For this review, take the finished solid that the model builds, in its own axes (mm). Face numbers are marked on the shaded views. Coordinates: 2 decimals unless noted, no trailing zeros. Loops run counter-clockwise (first coordinate to the right, second up) from the corner with the lowest first, then second, coordinate; pieces in that order, holes last. Notation, with made-up numbers: M -30.5,-21 L 1.5,-21 A28 ccw 1.5,1 Z; hole C 46.25,72.25 d5. An arc over 180 degrees is marked long. Put each result on its own line as item: value.
```python
from build123d import *
from OCP.BRepFilletAPI import BRepFilletAPI_MakeChamfer

# Parameters (mm, degrees)
SKETCH_1_R          = 2.05
EXTRUDE_1_DEPTH     = 10
CHAMFER_1_SIZE      = 4
CHAMFER_1_SIZE2     = 5.656854249
CHAMFER_1_SIZE2_2   = 3.265986324
SKETCH_2_R          = 12.5
CUT_EXTRUDE_1_DEPTH = 56.856960175
FILLET_1_R          = 2.5


with BuildPart() as part:
    # 草图1 → 凸台-拉伸1 (new, symmetric)
    with BuildSketch(Plane.XY):
        Polygon((-13.032253728, 10), (1.437002663, -44), (17.110272543, -44), (28, -10), (28, 10), align=None)
        Circle(SKETCH_1_R, mode=Mode.SUBTRACT)
        with Locations((20, 0)):
            Circle(SKETCH_1_R, mode=Mode.SUBTRACT)
        with Locations((9.110272543, -34)):
            Circle(SKETCH_1_R, mode=Mode.SUBTRACT)
    extrude(amount=EXTRUDE_1_DEPTH, both=True)

    # 倒角1: one chamfer whose edges measure the first distance from different faces: ONE call of the kernel's chamfer builder (chamfer() names one face for all edges)
    chamfer_1_edges_1 = [part.edges().sort_by_distance(p)[0] for p in [
        (1.437002663, -44, 0),
    ]]
    chamfer_1_side_1 = [part.faces().sort_by_distance(p)[0] for p in [
        (-5.797625533, -17, 0),
    ]]
    chamfer_1_edges_2 = [part.edges().sort_by_distance(p)[0] for p in [
        (-13.032253728, 10, 0),
    ]]
    chamfer_1_side_2 = [part.faces().sort_by_distance(p)[0] for p in [
        (-5.797625533, -17, 0),
    ]]
    chamfer_1_edges_3 = [part.edges().sort_by_distance(p)[0] for p in [
        (28, 10, 0),
    ]]
    chamfer_1 = BRepFilletAPI_MakeChamfer(part.part.solid().wrapped)
    for e in chamfer_1_edges_1:
        chamfer_1.Add(CHAMFER_1_SIZE, CHAMFER_1_SIZE2, e.wrapped, chamfer_1_side_1[0].wrapped)  # the first distance lies on this face
    for e in chamfer_1_edges_2:
        chamfer_1.Add(CHAMFER_1_SIZE, CHAMFER_1_SIZE2_2, e.wrapped, chamfer_1_side_2[0].wrapped)  # the first distance lies on this face
    for e in chamfer_1_edges_3:
        chamfer_1.Add(CHAMFER_1_SIZE, e.wrapped)
    add(Compound.cast(chamfer_1.Shape()), mode=Mode.REPLACE)

    # 草图2 → 切除-拉伸1 (cut, through all)
    with BuildSketch(Plane.XY.offset(10)):
        with Locations((29.991739345, -25.62060001)):
            Circle(SKETCH_2_R)
    extrude(amount=-CUT_EXTRUDE_1_DEPTH, mode=Mode.SUBTRACT)

    # 圆角1
    fillet_1_edges = [part.edges().sort_by_distance(p)[0] for p in [
        (-9.766267405, 10, 0),
        (24, 10, 0),
        (28, 6, 0),
        (0.401726482, -40.136296695, 0),
        (-11.996977548, 6.136296695, 0),
        (7.093856912, -44, 0),
        (26.873983288, -13.515658987, 0),
        (20.421472383, -33.661743602, 0),
        (17.110272543, -44, 0),
        (28, -10, 0),
    ]]
    fillet(fillet_1_edges, radius=FILLET_1_R)


solid = part.part
```
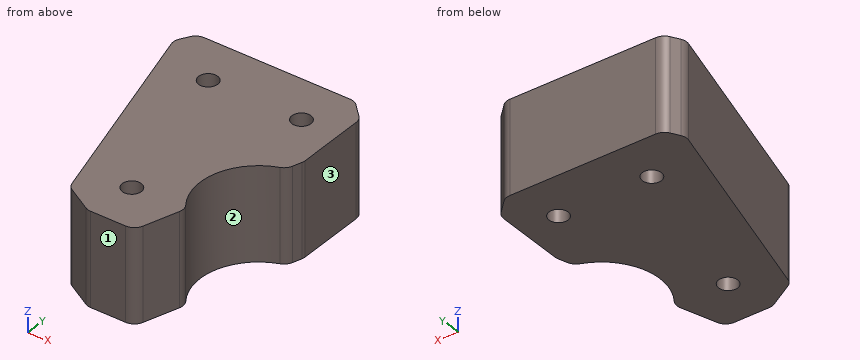
(1) Add section A-A (z = -2.25). Write out the cut boundary in (x, y), plus the area to 3 significant figures.
Determined:
outline: M -11.73,5.14 L 0.13,-39.14 A2.5 ccw 1.3,-40.65 L 6.51,-43.67 A2.5 ccw 7.76,-44 L 15.29,-44 A2.5 ccw 17.67,-42.26 L 20.02,-34.9 A2.5 ccw 19.7,-32.72 A12.5 cw 25.74,-13.87 A2.5 ccw 27.27,-12.28 L 27.88,-10.37 A2.5 ccw 28,-9.61 L 28,4.96 A2.5 ccw 27.27,6.73 L 24.73,9.27 A2.5 ccw 22.96,10 L -8.32,10 A2.5 ccw -10.49,8.75 L -11.48,7.03 A2.5 ccw Z; hole C 0,0 d4.1; hole C 9.11,-34 d4.1; hole C 20,0 d4.1
area: 1,490 mm^2
(2) Add section B-B (y = -1). Write out the cut boundary in (x, z).
Determined:
outline: M -10.08,-10 L -1.79,-10 L -1.79,10 L -10.08,10 Z; M 1.79,-10 L 18.21,-10 L 18.21,10 L 1.79,10 Z; M 21.79,-10 L 28,-10 L 28,10 L 21.79,10 Z
(3) Wall thickness on line 1 along Y through (x, z) = (9, -0.75); line 2 along X through (y, z) = (1, -6.75); line 3 along Y through (x, z) = (3, -3.5): over which ranges is each line inside the solid? List them lowest first. Write a range as [from, to].
Determined:
line 1: y = [-44, -36.05], [-31.95, 10]
line 2: x = [-10.62, -1.79], [1.79, 18.21], [21.79, 28]
line 3: y = [-41.64, 10]
(4) Draft analysis for pull direction Y (two halves, no side actions). For the marked faces 1, 2 and 3, state which applies: +Y half, -Y half, draft (parallel to the pull), parting line (faces both ways), or undercut.
Determined:
face 1: -Y half
face 2: undercut
face 3: draft
(5) Add section C-C (x = 9). Write out the cut boundary in (y, z).
Determined:
outline: M -44,-10 L -36.05,-10 L -36.05,10 L -44,10 Z; M -31.95,-10 L 10,-10 L 10,10 L -31.95,10 Z
(6) Add section D-D (y = -34). Write out the cut boundary in (x, z), plus the area to 3 significant figures.
Determined:
outline: M -1.24,-10 L 7.06,-10 L 7.06,10 L -1.24,10 Z; M 11.16,-10 L 20.14,-10 L 20.14,10 L 11.16,10 Z
area: 346 mm^2
(7) For pin 1 (1.5 mm diameter, centred on y = -18, z = -3.5, fed in from -X); pin 2 (1.5 mm diameter, centred on y = -14, z = 8, fed in from +X); pin 3 (8 mm diameter, centred on y = -20, z = 2, fed in from +X), all flat-tipped, find the tip position at first contact; note any pin that passes through.
Determined:
pin 1: stops at x = -5.73
pin 2: stops at x = 26.69
pin 3: stops at x = 22.01
